Read the model definition and answer for the solid it produces. Units are mm, in the model's axes. Round coordinates to 2 decimals unless told otherwise and drop trailing zeros. Put each result on its own line as item: value. Start each with the question number.
Q1. Find the intervals of material crossed by line 1 along Z through (x, y) = (0, -6); line 2 along X through (y, z) = (1.5, 19); line 3 along Y through (x, z) = (-2, 127), in increasing order. Write a range as from..to.
Q2. For a pull along Z with two mould halves and no side action, classify faces 1 (the face through (11.547, -4.788, 544.518)), 2 (the face through (0, 0, 1074)), 3 (the face through (0, 0, 0)) as pulls with the +Z half, pulls with the -Z half, needs draft (parallel to the pull), parting line crosses it, or undercut.
Q3. Each of these flat-tipped pins is pushed along its axis until it touches: pin 1 Ø1.3 at (y, z) = (13.5, 1067.5) entering from +X; pin 2 Ø8 at (x, z) = (-7, 752) entering from +Y; pin 3 Ø4 at (y, z) = (5.5, 947) entering from -X; pin 4 Ø1.4 at (x, y) = (1, 13.5) entering from -Z. Where does it stop, or does it pass through?
from build123d import *

# Parameters (mm, degrees)
SKETCH1_R           = 12.5
BOSS_EXTRUDE1_DEPTH = 537
BOSS_EXTRUDE2_DEPTH = 30
CIRPATTERN1_COUNT   = 4
SKETCH4_R           = 3
CUT_EXTRUDE1_DEPTH  = 538.418831081


# Read off the part's stored shape, not the designer's step: Mirror1
with BuildPart() as part:
    # Sketch1 → Boss-Extrude1 (new body)
    with BuildSketch(Plane.XY):
        Circle(SKETCH1_R)
    extrude(amount=BOSS_EXTRUDE1_DEPTH)

    # Sketch3 → Boss-Extrude2 (add)
    with BuildSketch(Plane(origin=(0, 0, 0), x_dir=(-1, 0, 0), z_dir=(0, 0, -1))):
        with BuildLine():
            Line((-2.5, 14.790199458), (-2.5, 12.247448714))
            ThreePointArc((-2.5, 12.247448714), (0, 12.5), (2.5, 12.247448714))
            Line((2.5, 12.247448714), (2.5, 14.790199458))
            ThreePointArc((2.5, 14.790199458), (0, 15), (-2.5, 14.790199458))
        make_face()
    boss_extrude2 = extrude(amount=-BOSS_EXTRUDE2_DEPTH)

    # CirPattern1: Boss-Extrude2 ×4 about axis
    cirpattern1_axis = Axis((0, 0, 0), (0, 0, 1))
    for i in range(1, CIRPATTERN1_COUNT):
        add(boss_extrude2.rotate(cirpattern1_axis, i * 360 / CIRPATTERN1_COUNT))

    # Sketch4 → Cut-Extrude1 (cut, symmetric)
    with BuildSketch(Plane(origin=(0, 0, 0), x_dir=(1, 0, 0), z_dir=(0, 1, 0))):
        with Locations(Location((0, -19, 0), (0, 0, 213.557309762))):
            Circle(SKETCH4_R)
    extrude(amount=CUT_EXTRUDE1_DEPTH, both=True, mode=Mode.SUBTRACT)

    # Mirror1: part across plane


with BuildPart() as part_1:
    add(part.part)
    add(part.part.mirror(Plane.XY.offset(537)))


solid = part_1.part
Findings:
1. line 1: 0..16, 22..1052, 1058..1074
1. line 2: -14.92..-3, 3..14.92
1. line 3: -12.34..12.34
2. face 1: undercut
2. face 2: pulls with the +Z half
2. face 3: pulls with the -Z half
3. pin 1: x = 2.5
3. pin 2: y = 12.13
3. pin 3: x = -12
3. pin 4: z = 0
